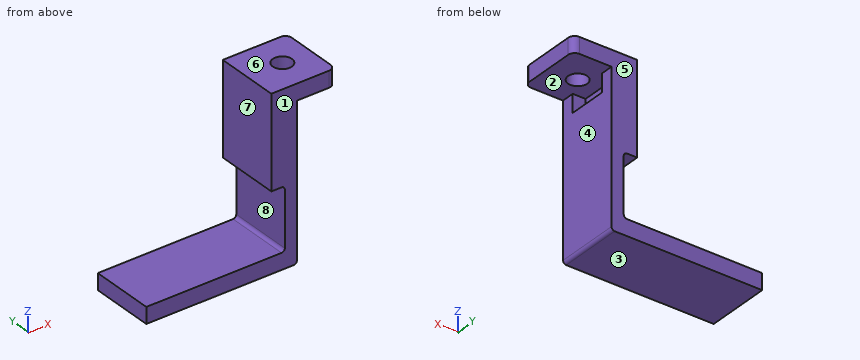
```python
from build123d import *

# Parameters (mm, degrees)
EXTRUDE_1_DEPTH     = 10
SKETCH_2_R          = 1.5
CUT_EXTRUDE_1_DEPTH = 10
FILLET_1_R          = 0.5
FILLET_2_R          = 0.5
FILLET_3_R          = 1
SKETCH_3_W          = 2.8
SKETCH_3_H          = 6
CUT_EXTRUDE_2_DEPTH = 2


with BuildPart() as part:
    # 草图1 → 凸台-拉伸1 (new body)
    with BuildSketch(Plane(origin=(0, 0, 0), x_dir=(1, 0, 0), z_dir=(0, 1, 0))):
        Polygon((0, 0), (10, 0), (10, 2.5), (4, 2.5), (4, 26.4), (-19.5, 26.4), (-19.5, 23.9), (2.1, 23.9), (2.1, 14.3), (0, 14.3), align=None)
    extrude(amount=EXTRUDE_1_DEPTH)

    # 草图2 → 切除-拉伸1 (cut)
    with BuildSketch(Plane(origin=(0, 0, -2.5), x_dir=(-1, 0, 0), z_dir=(0, 0, -1))):
        with Locations((-5.5, 5)):
            Circle(SKETCH_2_R)
    extrude(amount=-CUT_EXTRUDE_1_DEPTH, mode=Mode.SUBTRACT)

    # 圆角1
    fillet_1_edges = [part.edges().sort_by_distance(p)[0] for p in [
        (2.1, 5, -23.9),
        (4, 5, -26.4),
    ]]
    fillet(fillet_1_edges, radius=FILLET_1_R)

    # 圆角2
    fillet_2_edges = [part.edges().sort_by_distance(p)[0] for p in [
        (2.1, 5, -14.3),
    ]]
    fillet(fillet_2_edges, radius=FILLET_2_R)

    # 圆角3
    fillet_3_edges = [part.edges().sort_by_distance(p)[0] for p in [
        (10, 10, -1.25),
        (10, 0, -1.25),
    ]]
    fillet(fillet_3_edges, radius=FILLET_3_R)

    # 草图3 → 切除-拉伸2 (cut)
    with BuildSketch(Plane(origin=(4, 0, 0), x_dir=(0, 0, -1), z_dir=(1, 0, 0))):
        with Locations((3.9, 5)):
            Rectangle(SKETCH_3_W, SKETCH_3_H)
    extrude(amount=-CUT_EXTRUDE_2_DEPTH, mode=Mode.SUBTRACT)


solid = part.part
```
Read the model definition and answer for the solid it produces. Units are mm, in the model's axes. Face numbers are marked on the shaded views. A direction names the side the tool comes from. Round coordinates to 2 decimals unless told otherwise and drop trailing zeros. Write each loop counter-clockwise with the first axis right and the second up, starting at its lowest first coordinate (ties: lowest second). Pieces come first, ordered by that corner, then holes. Notation, with made-up numbers: M -16,-27 L 0,-27 A25 cw 0,9 Z; hole C -5.75,-20 d5. An arc over 180 degrees is marked long. One line per item, written item: value.
Q1. Flat-ended cylindrical pins translate along their axes: pin 1 Ø5 at (x, y) = (-1, 3.5) entering from +Z; pin 2 Ø5 at (y, z) = (4.5, -10) entering from -X; pin 3 Ø1 at (x, y) = (-3, 2.5) entering from +Z; pin 4 Ø1.5 at (y, z) = (6, -9.5) entering from +X. Find the tip coordinate at first contact, or state that the pin passes through.
Data:
pin 1: z = 0
pin 2: x = 0
pin 3: z = -23.9
pin 4: x = 4
Q2. Find section A-A on x = 5.5. Write down the section's boundary in (y, z).
Data:
outline: M 0,-2.5 L 3.5,-2.5 L 3.5,0 L 0,0 Z; M 6.5,-2.5 L 10,-2.5 L 10,0 L 6.5,0 Z
Q3. Straight lines are drawn through the part: line 1 (Y direction, x = 5.5, z = -1.95); line 2 (Z direction, x = 0.5, y = 1.5); line 3 (Z direction, x = -12.25, y = 4.75). For each, find the intervals that lie inside material, in ascending order. Write a range as [from, to].
Data:
line 1: [0, 3.5], [6.5, 10]
line 2: [-26.4, -23.9], [-14.3, 0]
line 3: [-26.4, -23.9]
Q4. Which of the six approach directions +Z, -Z, +X, -X, +Y, -Y give full straight-line access (tool end or side, diameter ignored) to the marked faces 4, 5, 6, 7 and 8?
Data:
face 4: -Z, +X, +Y, -Y
face 5: +Z, -Z, +X, -X, +Y
face 6: +Z, +X, -X, +Y, -Y
face 7: +Z, -X, +Y, -Y
face 8: -X, +Y, -Y
Q5. Find section D-D on y = 3. Write down the section's boundary in (x, z).
Data:
outline: M -19.5,-26.4 L 3.5,-26.4 A0.5 ccw 4,-25.9 L 4,-5.3 L 2,-5.3 L 2,-2.5 L 10,-2.5 L 10,0 L 0,0 L 0,-14.3 L 1.6,-14.3 A0.5 cw 2.1,-14.8 L 2.1,-23.4 A0.5 cw 1.6,-23.9 L -19.5,-23.9 Z
Q6. For a pull along Y with two mould halves and no side action, classify the marked faces 1, 2 and 3 as +Y half, -Y half, draft (parallel to the pull), parting line (faces both ways), or undercut.
Data:
face 1: -Y half
face 2: undercut
face 3: draft
Q7. Find section B-B on y = 5. Write down the section's boundary in (x, z).
Data:
outline: M -19.5,-26.4 L 3.5,-26.4 A0.5 ccw 4,-25.9 L 4,-5.3 L 2,-5.3 L 2,-2.5 L 4,-2.5 L 4,0 L 0,0 L 0,-14.3 L 1.6,-14.3 A0.5 cw 2.1,-14.8 L 2.1,-23.4 A0.5 cw 1.6,-23.9 L -19.5,-23.9 Z; M 7,-2.5 L 10,-2.5 L 10,0 L 7,0 Z
Q8. Find section C-C on z = -4.5. Write down the section's boundary in (x, y).
Data:
outline: M 0,0 L 4,0 L 4,2 L 2,2 L 2,8 L 4,8 L 4,10 L 0,10 Z
